The listing builds one solid part. Answer for the finished solid, in the listing's coordinates (mm). A direction names the side the tool comes from. Coordinates: 2 decimals unless noted, no trailing zeros. Order: outer loops, then holes, each group sorted by start corner. A loop starts at its lowest first (then second) coordinate and runs counter-clockwise, first axis right, second up.
```python
from build123d import *

# Parameters (mm, degrees)
SKETCH001_R   = 4
SKETCH001_R_2 = 2.5
POCKET_DEPTH  = 38.321


with BuildPart() as part:
    # Sketch → Revolution (revolve)
    with BuildSketch(Plane.XZ):
        Polygon((0, 0), (0, 39.63), (2.13, 39.63), (2.13, 37.5), (33.82, 37.5), (38.32, 37.2), (38.32, 35.7), (2.13, 35.7), (2.13, 0), align=None)
    revolve(axis=Axis((0, 0, 0), (1, 0, 0)))

    # Sketch001 (on Face1 of Revolution) → Pocket (cut, through all)
    with BuildSketch(Plane(origin=(0, 0, 0), x_dir=(0, 0, -1), z_dir=(-1, 0, 0))):
        Circle(SKETCH001_R)
        with Locations((0, 18.5)):
            Circle(SKETCH001_R_2)
        with Locations((0, -18.5)):
            Circle(SKETCH001_R_2)
        with Locations((21.75, -18.5)):
            Circle(SKETCH001_R)
    extrude(amount=-POCKET_DEPTH, mode=Mode.SUBTRACT)


solid = part.part
```
(1) Find section A-A (z = 0). Write down the section's boundary in (x, y), and give its area (3 significant figures).
(2) Each of these flat-tipped pins is pushed along its axis until it touches: pin 1 Ø2 at (x, y) = (9.5, 22.5) entering from +Z; pin 2 Ø12 at (x, y) = (21.5, 23.5) entering from +Z; pin 3 Ø21.5 at (y, z) = (-14, 0) entering from +X; pin 4 Ø8 at (y, z) = (30.5, -13) entering from +X. Where does it stop, or does it pass through?
(3) For faces 1 (the face through (1.1, 15.8, -18.8)), 2 (the face through (18.2, -37.18, -4.88)), determine the directions among +Z, -Z, +X, -X, +Y, -Y from which every point of the face is accessible in a straight line to the end or side of a thin tool.
(4) Consider line 1 (Y direction, x = 1.15, z = 0); line 2 (Y direction, x = 24.5, z = 0); line 3 (X direction, y = 6.5, z = -18). Determine where each line is inside the solid, lowest interval first.
(5) Find section B-B (x = 32.5). Write down the section's boundary in (y, z).
(6) Find section C-C (y = 18.5). Give the number of separate pieces and of enclosed holes in the cut face, and give its area (3 significant figures).
(7) The mould has two halves that part along Z. Classify faces 3 (the face through (38.32, -14, -33.2)), 4 (the face through (1.08, 24.11, -31.45)), 5 (the face through (19.972, -1.57, -35.665)): released by +Z, released by -Z, zero draft, split by the parting line, or undercut.
Findings below:
1. outline: (0, -39.63) - (2.13, -39.63) - (2.13, -37.5) - (33.82, -37.5) - (38.32, -37.2) - (38.32, -35.7) - (2.13, -35.7) - (2.13, -21) - (0, -21) - close; (0, -16) - (2.13, -16) - (2.13, -4) - (0, -4) - close; (0, 4) - (2.13, 4) - (2.13, 16) - (0, 16) - close; (0, 21) - (2.13, 21) - (2.13, 35.7) - (38.32, 35.7) - (38.32, 37.2) - (33.82, 37.5) - (2.13, 37.5) - (2.13, 39.63) - (0, 39.63) - close
1. area: 259 mm2
2. pin 1: stops at z = 30.72
2. pin 2: stops at z = 33.17
2. pin 3: stops at x = 2.13
2. pin 4: stops at x = 38.32
3. face 1: +X, -X
3. face 2: +X
4. line 1: y = -39.63 to -21, -16 to -4, 4 to 16, 21 to 39.63
4. line 2: y = -37.5 to -35.7, 35.7 to 37.5
4. line 3: x = 0 to 2.13
5. outline: circle Ø75 at (0, 0); hole circle Ø71.4 at (0, 0)
6. separate pieces: 3
6. enclosed holes: 0
6. area: 271 mm2
7. face 3: zero draft
7. face 4: split by the parting line
7. face 5: undercut
